```python
from build123d import *

# Parameters (mm, degrees)
SKETCH1_R           = 75
BOSS_EXTRUDE1_DEPTH = 3.175
CUT_EXTRUDE1_DEPTH  = 3.175
SKETCH3_R           = 1.5875
CUT_EXTRUDE2_DEPTH  = 3.175
SKETCH4_R           = 27.051
CUT_EXTRUDE3_DEPTH  = 3.175
CUT_EXTRUDE4_DEPTH  = 3.175


with BuildPart() as part:
    # Sketch1 → Boss-Extrude1 (new body)
    with BuildSketch(Plane(origin=(0, 0, 0), x_dir=(1, 0, 0), z_dir=(0, 1, 0))):
        Circle(SKETCH1_R)
    extrude(amount=BOSS_EXTRUDE1_DEPTH)

    # Sketch2 → Cut-Extrude1 (cut)
    with BuildSketch(Plane(origin=(0, 3.175, 0), x_dir=(1, 0, 0), z_dir=(0, 1, 0))):
        with BuildLine():
            Line((-56.262005909, -49.594220339), (56.262005909, -49.594220339))
            ThreePointArc((56.262005909, -49.594220339), (0, -75), (-56.262005909, -49.594220339))
        make_face()
        with BuildLine():
            Line((-56.262005909, 49.594220339), (56.262005909, 49.594220339))
            ThreePointArc((56.262005909, 49.594220339), (0, 75), (-56.262005909, 49.594220339))
        make_face()
    extrude(amount=-CUT_EXTRUDE1_DEPTH, mode=Mode.SUBTRACT)

    # Sketch3 → Cut-Extrude2 (cut)
    with BuildSketch(Plane(origin=(0, 3.175, 0), x_dir=(1, 0, 0), z_dir=(0, 1, 0))):
        with Locations((-52.180304588, 44.729838125)):
            Circle(SKETCH3_R)
        with Locations((-19.05, 44.729838125)):
            Circle(SKETCH3_R)
        with Locations((19.05, 44.729838125)):
            Circle(SKETCH3_R)
        with Locations((52.180304588, 44.729838125)):
            Circle(SKETCH3_R)
        with Locations((52.180304588, -44.729838125)):
            Circle(SKETCH3_R)
        with Locations((19.05, -44.729838125)):
            Circle(SKETCH3_R)
        with Locations((-19.05, -44.729838125)):
            Circle(SKETCH3_R)
        with Locations((-52.180304588, -44.729838125)):
            Circle(SKETCH3_R)
    extrude(amount=-CUT_EXTRUDE2_DEPTH, mode=Mode.SUBTRACT)

    # Sketch4 → Cut-Extrude3 (cut)
    with BuildSketch(Plane(origin=(0, 3.175, 0), x_dir=(1, 0, 0), z_dir=(0, 1, 0))):
        with BuildLine():
            Line((-47.315937317, 44.741895283), (-23.177806764, 24.050282215))
            ThreePointArc((-23.177806764, 24.050282215), (-19.742091457, 26.942097653), (-15.949506316, 29.346891646))
            Line((-15.949506316, 29.346891646), (-20.527078848, 40.095137229))
            ThreePointArc((-20.527078848, 40.095137229), (-22.980849122, 41.864416778), (-23.914367271, 44.741895283))
            Line((-23.914367271, 44.741895283), (-47.315937317, 44.741895283))
        make_face()
        with BuildLine():
            ThreePointArc((10.107278818, 31.835039122), (0, 33.401), (-10.107278818, 31.835039122))
            Line((-10.107278818, 31.835039122), (-14.68485135, 42.583284705))
            ThreePointArc((-14.68485135, 42.583284705), (-14.312069768, 43.627916425), (-14.185617786, 44.729838125))
            Line((-14.185617786, 44.729838125), (14.185617786, 44.729838125))
            ThreePointArc((14.185617786, 44.729838125), (14.312069768, 43.627916425), (14.68485135, 42.583284705))
            Line((14.68485135, 42.583284705), (10.107278818, 31.835039122))
        make_face()
        with BuildLine():
            ThreePointArc((15.949506316, 29.346891646), (19.742091457, 26.942097653), (23.177806764, 24.050282215))
            Line((23.177806764, 24.050282215), (47.315937317, 44.741895283))
            Line((47.315937317, 44.741895283), (23.914382214, 44.729838125))
            ThreePointArc((23.914382214, 44.729838125), (22.977294896, 41.859547352), (20.527078848, 40.095137229))
            Line((20.527078848, 40.095137229), (15.949506316, 29.346891646))
        make_face()
        Circle(SKETCH4_R)
        with BuildLine():
            Line((-23.177806764, -24.050282215), (-47.315937317, -44.741895283))
            Line((-47.315937317, -44.741895283), (-23.914382214, -44.729838125))
            ThreePointArc((-23.914382214, -44.729838125), (-22.977294896, -41.859547352), (-20.527078848, -40.095137229))
            Line((-20.527078848, -40.095137229), (-15.949506316, -29.346891646))
            ThreePointArc((-15.949506316, -29.346891646), (-19.742091457, -26.942097653), (-23.177806764, -24.050282215))
        make_face()
        with BuildLine():
            ThreePointArc((-10.107278818, -31.835039122), (0, -33.401), (10.107278818, -31.835039122))
            Line((10.107278818, -31.835039122), (14.68485135, -42.583284705))
            ThreePointArc((14.68485135, -42.583284705), (14.312069768, -43.627916425), (14.185617786, -44.729838125))
            Line((14.185617786, -44.729838125), (-14.185617786, -44.729838125))
            ThreePointArc((-14.185617786, -44.729838125), (-14.312069768, -43.627916425), (-14.68485135, -42.583284705))
            Line((-14.68485135, -42.583284705), (-10.107278818, -31.835039122))
        make_face()
        with BuildLine():
            ThreePointArc((23.177806764, -24.050282215), (19.742091457, -26.942097653), (15.949506316, -29.346891646))
            Line((15.949506316, -29.346891646), (20.527078848, -40.095137229))
            ThreePointArc((20.527078848, -40.095137229), (22.977294896, -41.859547352), (23.914382214, -44.729838125))
            Line((23.914382214, -44.729838125), (47.315937317, -44.741895283))
            Line((47.315937317, -44.741895283), (23.177806764, -24.050282215))
        make_face()
    extrude(amount=-CUT_EXTRUDE3_DEPTH, mode=Mode.SUBTRACT)

    # Sketch5 → Cut-Extrude4 (cut)
    with BuildSketch(Plane(origin=(0, 3.175, 0), x_dir=(1, 0, 0), z_dir=(0, 1, 0))):
        with BuildLine():
            Line((58.957481542, 46.357473725), (27.31053772, 19.229179141))
            ThreePointArc((27.31053772, 19.229179141), (33.401, 0), (27.31053772, -19.229179141))
            Line((27.31053772, -19.229179141), (58.957481542, -46.357473725))
            ThreePointArc((58.957481542, -46.357473725), (75, 0), (58.957481542, 46.357473725))
        make_face()
    extrude(amount=-CUT_EXTRUDE4_DEPTH, mode=Mode.SUBTRACT)


solid = part.part
```
Source: CAD feature listing. Evaluate the final solid. Frame: model axes, mm. A direction names the side the tool comes from. Coordinates: 2 decimals unless noted, no trailing zeros. Write each loop counter-clockwise with the first axis right and the second up, starting at its lowest first coordinate (ties: lowest second). Pieces come first, ordered by that corner, then holes. Notation, with made-up numbers: (-31, 11) - (2, 11) arc R19 ccw to (2, 17) - close; hole circle Ø9 at (-2, 1). An arc over 180 degrees is marked (long way). Answer as a JSON object with one key per item and string values.
Q1. Section query A-A, the plane x = 0. Output: boundary loops of the cut face in (y, z) (3 decimals), plus the area to 3 significant figures.
Ans:
{"outline": "(0, -49.594) - (3.175, -49.594) - (3.175, -44.73) - (0, -44.73) - close; (0, -33.401) - (3.175, -33.401) - (3.175, -27.051) - (0, -27.051) - close; (0, 27.051) - (3.175, 27.051) - (3.175, 33.401) - (0, 33.401) - close; (0, 44.73) - (3.175, 44.73) - (3.175, 49.594) - (0, 49.594) - close", "area": "71.2 mm2"}
Q2. Material intervals for line 1 (Z direction, x = -19.05, y = 1.7); line 2 (X direction, y = 0.95, z = -34); line 3 (Z direction, x = -16.5, y = 1.85), sorted ascending. Write a range as [from, to].
Ans:
{"line 1": "z = [-49.59, -46.32], [-43.14, -36.63], [-27.44, -19.21], [19.21, 27.44], [36.63, 43.14], [46.32, 49.59]", "line 2": "x = [-66.85, -34.78], [-17.93, -11.03], [11.03, 17.93], [34.78, 44.54]", "line 3": "z = [-49.59, -30.64], [-29.04, -21.44], [21.44, 29.04], [30.64, 49.59]"}
Q3. Draft query along Z for faces 4 (the cylindrical face through (25.8, 1.61, -8.13)), 5 (the flat face through (-1, 2, -49.594)), 6 (the flat face through (-1, 2, 49.594)). Return one class per face: released by +Z, released by -Z, zero draft, split by the parting line, or undercut.
Ans:
{"face 4": "undercut", "face 5": "released by -Z", "face 6": "released by +Z"}
Q4. Section query B-B, the plane z = 0. Output: boundary loops of the cut face in (x, y) (3 decimals).
Ans:
{"outline": "(-75, 0) - (-27.051, 0) - (-27.051, 3.175) - (-75, 3.175) - close; (27.051, 0) - (33.401, 0) - (33.401, 3.175) - (27.051, 3.175) - close"}
Q5. First-contact query: pin 1 Ø3 at (x, z) = (-52.18, -44.73) entering from +Y. Flat tip, straight axial feed; report the tip coordinate or a pass-through.
Ans:
{"pin 1": "passes through"}
Q6. Section query D-D, the plane y = 0.6. State how many separate pieces and enclosed holes the cut face has, plus the area to 3 significant figures.
Ans:
{"separate pieces": "1", "enclosed holes": "15", "area": "6,520 mm2"}
Q7. Section query C-C, the plane x = -38.5. Output: boundary loops of the cut face in (y, z) (3 decimals), plus the area to 3 significant figures.
Ans:
{"outline": "(0, -49.594) - (3.175, -49.594) - (3.175, -44.742) - (0, -44.742) - close; (0, -37.185) - (3.175, -37.185) - (3.175, 37.185) - (0, 37.185) - close; (0, 44.737) - (3.175, 44.737) - (3.175, 49.594) - (0, 49.594) - close", "area": "267 mm2"}
Q8. Set-up query: faces 1 (the flat face through (42.91, 1.61, 32.6)), 2 (the cylindrical face through (57.651, 1.565, -47.972)), 3 (the flat face through (12.364, 1.61, 37.134)). Return all of +Z, -Z, +X, -X, +Y, -Y with unobstructed straight access to the full face (end or side cutting, diameter ignored); none if empty.
Ans:
{"face 1": "+X, +Y, -Y", "face 2": "-Z, +X, +Y, -Y", "face 3": "+Y, -Y"}
